Design review of the part shown in the three views and the two pictorial views. Dimensions are in mm from the part's minimum x, y and z. Round coordinates to 2 decimals unless told otherwise and drop trailing zeros. Order: outer loops, then holes, each group sorted by start corner. A loop starts at its lowest first (then second) coordinate and runs counter-clockwise, first axis right, second up.
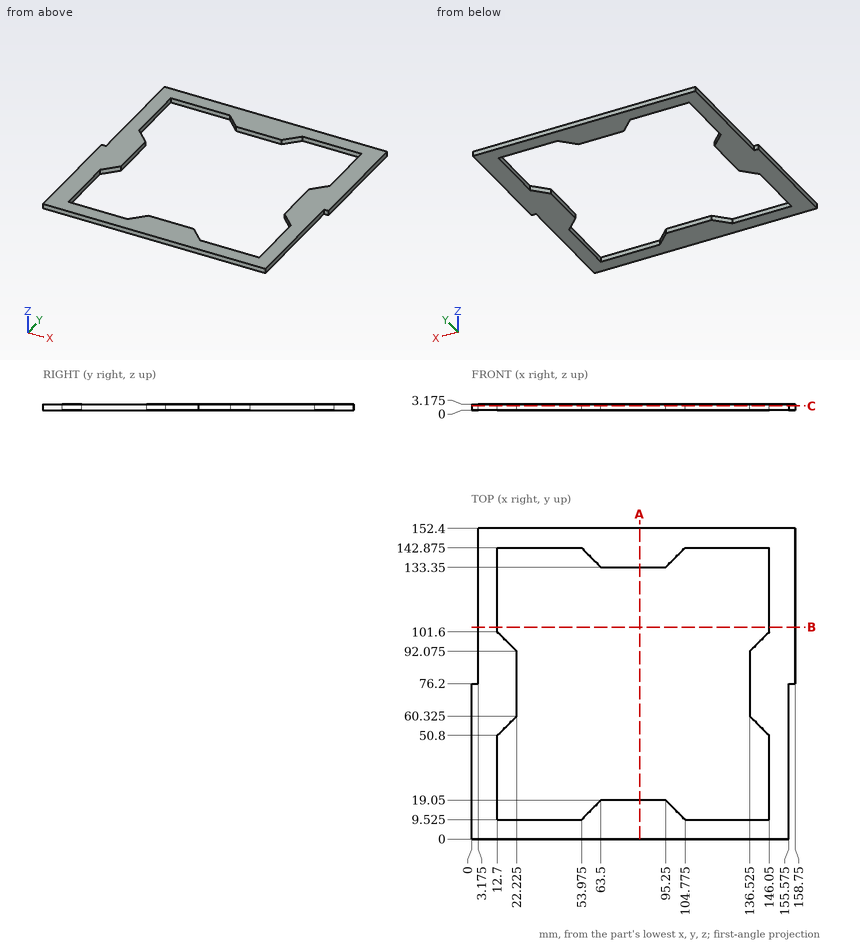
(1) Add section A-A on x = 82.5. Give the boundary of the cut face in (y, z) (3 decimals), plus the area to 3 significant figures.
(2) Add section B-B on y = 104. Give the boundary of the cut face in (x, z) (3 decimals), plus the area to 3 significant figures.
(3) Wall thickness on L1, parallel to X at y = 46, z = 1.85 (3 decimals); L2, parallel to X at y = 124, z = 2.7 (3 decimals); L3, parallel to Y at x = 129, z = 1.85 (3 decimals): over which ranges is each line inside the solid? List them lowest first.
(4) Clearance check with flat-ended pins moving along their axes: P1, Ø1.6, axis at y = 36, z = 2.5, coming from the +X side (3 decimals); P2, Ø5, axis at x = 141, y = 92.5, coming from the -Z side; P3, Ø1, axis at y = 77.5, z = 1, coming from the -X side (3 decimals). State where each tip first meets the part, or that it passes through.
(5) Add section C-C on z = 2.3. Give the boundary of the cut face in (x, y) (3 decimals).
Here are the results:
1. outline: (0, 0) - (19.05, 0) - (19.05, 3.175) - (0, 3.175) - close; (133.35, 0) - (152.4, 0) - (152.4, 3.175) - (133.35, 3.175) - close
1. area: 121 mm2
2. outline: (3.175, 0) - (12.7, 0) - (12.7, 3.175) - (3.175, 3.175) - close; (146.05, 0) - (158.75, 0) - (158.75, 3.175) - (146.05, 3.175) - close
2. area: 70.6 mm2
3. L1: x = 0 to 12.7, 146.05 to 155.575
3. L2: x = 3.175 to 12.7, 146.05 to 158.75
3. L3: y = 0 to 9.525, 142.875 to 152.4
4. P1: stops at x = 155.575
4. P2: stops at z = 0
4. P3: stops at x = 3.175
5. outline: (0, 0) - (155.575, 0) - (155.575, 76.2) - (158.75, 76.2) - (158.75, 152.4) - (3.175, 152.4) - (3.175, 76.2) - (0, 76.2) - close; hole (12.7, 9.525) - (53.975, 9.525) - (63.5, 19.05) - (95.25, 19.05) - (104.775, 9.525) - (146.05, 9.525) - (146.05, 50.8) - (136.525, 60.325) - (136.525, 92.075) - (146.05, 101.6) - (146.05, 142.875) - (104.775, 142.875) - (95.25, 133.35) - (63.5, 133.35) - (53.975, 142.875) - (12.7, 142.875) - (12.7, 101.6) - (22.225, 92.075) - (22.225, 60.325) - (12.7, 50.8) - close
